from build123d import *

# Parameters (mm, degrees)
CROQUIS1_W              = 38.1
CROQUIS1_H              = 6.31
SALIENTE_EXTRUIR1_DEPTH = 330.7
CROQUIS3_W              = 38.1
CROQUIS3_H              = 6.31
SALIENTE_EXTRUIR2_DEPTH = 658.79
CROQUIS4_R              = 6.35
CORTAR_EXTRUIR1_DEPTH   = 6.31


with BuildPart() as part:
    # Croquis1 → Saliente-Extruir1 (new body)
    with BuildSketch(Plane.XY):
        Rectangle(CROQUIS1_W, CROQUIS1_H)
    extrude(amount=SALIENTE_EXTRUIR1_DEPTH)

    # Croquis3 → Saliente-Extruir2 (add)
    with BuildSketch(Plane.XZ.offset(3.155)):
        with Locations((0, 3.155)):
            Rectangle(CROQUIS3_W, CROQUIS3_H)
    extrude(amount=-SALIENTE_EXTRUIR2_DEPTH)

    # Croquis4 → Cortar-Extruir1 (cut)
    with BuildSketch(Plane(origin=(0, -3.155, 0), x_dir=(-1, 0, 0), z_dir=(0, -1, 0))):
        with Locations(Location((0, -286.807795334, 0), (0, 0, 90))):
            Circle(CROQUIS4_R)
        with Locations(Location((0, -318.807795334, 0), (0, 0, 90))):
            Circle(CROQUIS4_R)
    extrude(amount=-CORTAR_EXTRUIR1_DEPTH, mode=Mode.SUBTRACT)


solid = part.part
Could you check a few things on this model? Use its own coordinates, in mm. A direction names the side the tool comes from. Coordinates: 2 decimals unless noted, no trailing zeros. Loops run counter-clockwise (first coordinate to the right, second up) from the corner with the lowest first, then second, coordinate; pieces in that order, holes last.
1. Imagine slicing it at B-B (y = 577). Please give me the cut outline in (x, z), and give its area (3 significant figures).
2. Imagine slicing it at C-C (z = 253). Please give me the cut outline in (x, y) (3 decimals).
3. For P1, Ø4, axis at x = 13.5, y = 318, coming from the +Z side; P2, Ø11.5, axis at x = 0, z = 286.81, coming from the -Y side, each with a flat end and sliding along its axis, tell me the tip position at first contact or that it passes through.
4. For faces 4 (the face through (0, -3.155, 163)), 5 (the face through (0, 3.155, 166)), which set-ups out of +Z, -Z, +X, -X, +Y, -Y let a thin tool reach every point of the face, with its end or its side?
5. I need wall thicknesses on L1, parallel to Z at x = 0, y = 113; L2, parallel to Y at x = -15, z = 309 (3 decimals). Which ranges of each line are inside material? Lowest first, please.
6. We'd pull the mould along X, two halves only. Please class faces 1 (the face through (19.05, 325, 5)), 2 (the face through (0, 325, 6.31)), 3 (the face through (0.28, -0.04, 325.15)): released by +X, released by -X, zero draft, split by the parting line, or undercut.
7. Imagine slicing it at A-A (x = 0). Please give me the cut outline in (y, z) (3 decimals).
Computed values:
1. outline: (-19.05, 0) - (19.05, 0) - (19.05, 6.31) - (-19.05, 6.31) - close
1. area: 240 mm2
2. outline: (-19.05, -3.155) - (19.05, -3.155) - (19.05, 3.155) - (-19.05, 3.155) - close
3. P1: stops at z = 6.31
3. P2: passes through
4. face 4: +Z, -Z, +X, -X, -Y
4. face 5: +Z, +X, -X, +Y
5. L1: z = 0 to 6.31
5. L2: y = -3.155 to 3.155
6. face 1: released by +X
6. face 2: zero draft
6. face 3: undercut
7. outline: (-3.155, 0) - (655.635, 0) - (655.635, 6.31) - (3.155, 6.31) - (3.155, 280.458) - (-3.155, 280.458) - close; (-3.155, 293.158) - (3.155, 293.158) - (3.155, 312.458) - (-3.155, 312.458) - close; (-3.155, 325.158) - (3.155, 325.158) - (3.155, 330.7) - (-3.155, 330.7) - close
